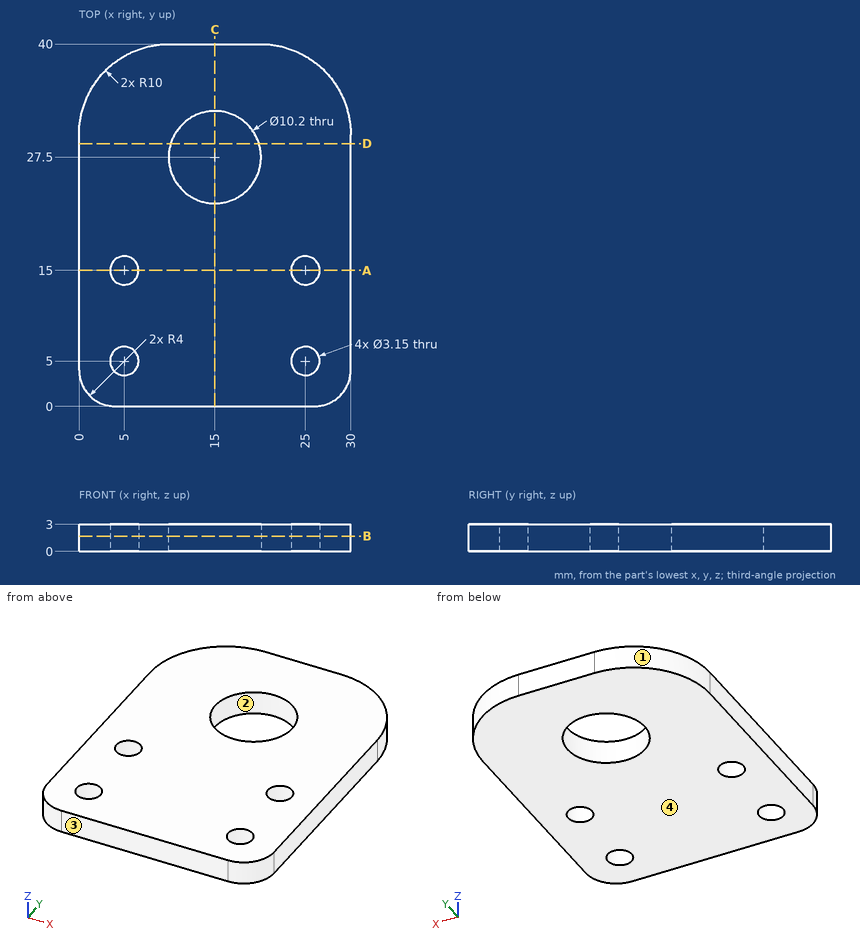
Answer from the drawing. Dimensions are ordinates in mm from the lowest x, y and z of the part. Round coordinates to 2 decimals unless told otherwise and drop trailing zeros. Write each loop counter-clockwise with the first axis right and the second up, starting at its lowest first coordinate (ties: lowest second). Pieces come first, ordered by that corner, then holes. Notation, with made-up numbers: (-36.75, 81.5) -> (-23.75, 81.5) arc R19 cw to (-23.75, 96.5) -> close; hole circle Ø2 at (18.5, 34.25). An arc over 180 degrees is marked (long way). Answer in a Markdown table with one row per item. Add a question column.
1) Find section A-A, the plane y = 15. Determine the outline of the cut face in (x, z) (3 decimals), and give its area (3 significant figures).
2) Consider line 1 (Y direction, x = 5, z = 0.9) (3 decimals); line 2 (X direction, y = 16, z = 0.95); line 3 (Y direction, x = 24.5, z = 2.5). Determine where each line is inside the solid, lowest interval first.
3) Given P1, Ø4, axis at x = 15.5, y = 26.5, coming from the -Z side (3 decimals), flat-ended and moving along its own axis, determine where the tip first touches the part or whether it passes through.
4) Determine the mould class of the marked faces 1, 2, 3 and 4 for opening direction Y: pulls with the +Y half, pulls with the -Y half, needs draft (parallel to the pull), parting line crosses it, or undercut.
5) Find section D-D, the plane y = 29. Determine the outline of the cut face in (x, z).
6) Find section C-C, the plane x = 15. Determine the outline of the cut face in (y, z), and give its area (3 significant figures).
7) Find section B-B, the plane z = 1.7. Determine the outline of the cut face in (x, y) (3 decimals).
Findings below:
| question | item | result |
|---|---|---|
| 1 | outline | (0, 0) -> (3.425, 0) -> (3.425, 3) -> (0, 3) -> close; (6.575, 0) -> (23.425, 0) -> (23.425, 3) -> (6.575, 3) -> close; (26.575, 0) -> (30, 0) -> (30, 3) -> (26.575, 3) -> close |
| 1 | area | 71.1 mm² |
| 2 | line 1 | 0 to 3.425, 6.575 to 13.425, 16.575 to 38.66 |
| 2 | line 2 | 0 to 3.78, 6.22 to 23.78, 26.22 to 30 |
| 2 | line 3 | 0 to 3.51, 6.49 to 13.51, 16.49 to 38.93 |
| 3 | P1 | through |
| 4 | face 1 | pulls with the +Y half |
| 4 | face 2 | undercut |
| 4 | face 3 | pulls with the -Y half |
| 4 | face 4 | needs draft |
| 5 | outline | (0, 0) -> (10.13, 0) -> (10.13, 3) -> (0, 3) -> close; (19.87, 0) -> (30, 0) -> (30, 3) -> (19.87, 3) -> close |
| 6 | outline | (0, 0) -> (22.4, 0) -> (22.4, 3) -> (0, 3) -> close; (32.6, 0) -> (40, 0) -> (40, 3) -> (32.6, 3) -> close |
| 6 | area | 89.4 mm² |
| 7 | outline | (0, 4) arc R4 ccw to (4, 0) -> (26, 0) arc R4 ccw to (30, 4) -> (30, 30) arc R10 ccw to (20, 40) -> (10, 40) arc R10 ccw to (0, 30) -> close; hole circle Ø3.15 at (5, 5); hole circle Ø3.15 at (5, 15); hole circle Ø10.2 at (15, 27.5); hole circle Ø3.15 at (25, 5); hole circle Ø3.15 at (25, 15) |
